```python
from build123d import *

# Parameters (mm, degrees)
ESQUISSE1_R                  = 5
BOSS_EXTRU_1_DEPTH           = 1280
ESQUISSE2_R                  = 15
BOSS_EXTRU_2_DEPTH           = 500
ESQUISSE3_R                  = 10
BOSS_EXTRU_3_DEPTH           = 400
CHANFREIN1_SIZE              = 10
CHANFREIN1_SIZE_2            = 43.314758743
ENL_V_MAT_EXTRU_1_DEPTH      = 1281.175769182
ENL_V_MAT_EXTRU_1_DEPTH_BACK = 1281.175769182
ESQUISSE4_R                  = 4
ESQUISSE5_R                  = 13
ESQUISSE5_R_2                = 9.409989574
BOSS_EXTRU_4_DEPTH           = 10
ESQUISSE7_R                  = 8
ESQUISSE7_R_2                = 4.592937417
BOSS_EXTRU_5_DEPTH           = 10
ESQUISSE6_R                  = 8
ESQUISSE6_R_2                = 4.579122691
BOSS_EXTRU_6_DEPTH           = 10
BOSS_EXTRU_7_START           = 720
BOSS_EXTRU_7_OUTLINE_R       = 13
BOSS_EXTRU_7_OUTLINE_R_2     = 10
BOSS_EXTRU_7_DEPTH           = 10
ESQUISSE8_R                  = 8
ESQUISSE8_R_2                = 4.5
BOSS_EXTRU_8_DEPTH           = 3


# Read off the part's stored shape, not the designer's step: Boss.-Extru.7
with BuildPart() as part:
    # Esquisse1 → Boss.-Extru.1 (new body)
    with BuildSketch(Plane(origin=(0, 0, 0), x_dir=(1, 0, 0), z_dir=(0, 1, 0))):
        with Locations(Location((0, 0, 0), (0, 0, 270))):
            Circle(ESQUISSE1_R)
    extrude(amount=BOSS_EXTRU_1_DEPTH)

    # Esquisse2 → Boss.-Extru.2 (add)
    with BuildSketch(Plane(origin=(0, 0, 0), x_dir=(1, 0, 0), z_dir=(0, 1, 0))):
        with Locations(Location((0, 0, 0), (0, 0, 270))):
            Circle(ESQUISSE2_R)
    extrude(amount=BOSS_EXTRU_2_DEPTH)

    # Esquisse3 → Boss.-Extru.3 (add)
    with BuildSketch(Plane(origin=(0, 500, 0), x_dir=(1, 0, 0), z_dir=(0, 1, 0))):
        with Locations(Location((0, 0, 0), (0, 0, 270))):
            Circle(ESQUISSE3_R)
    extrude(amount=BOSS_EXTRU_3_DEPTH)

    # Chanfrein1
    # the kernel refuses this chamfer: 43.314758743, 10 mm, written as the material it adds along each edge
    with BuildSketch(Plane(origin=(0, 500, 0), x_dir=(0, 0, 1), z_dir=(-1, 0, 0))) as chanfrein1_piece_1_section:
        Polygon((10 + CHANFREIN1_SIZE, 0), (10, CHANFREIN1_SIZE_2), (10, 0), align=None)
    chanfrein1_piece_1 = revolve(axis=Axis((0, 500, 0), (0, 1, 0)), mode=Mode.PRIVATE)
    chanfrein1_piece_1 = chanfrein1_piece_1 & Plane(origin=(0, 533.274352099, 0), x_dir=(0, 0, 1), z_dir=(0, -1, 0)) * Cylinder(15, 174, mode=Mode.PRIVATE)
    add(chanfrein1_piece_1)
    with BuildSketch(Plane(origin=(0, 900, 0), x_dir=(0, 0, 1), z_dir=(1, 0, 0))) as chanfrein1_piece_2_section:
        Polygon((5 + CHANFREIN1_SIZE, 0), (5, -CHANFREIN1_SIZE_2), (5, 0), align=None)
    chanfrein1_piece_2 = revolve(axis=Axis((0, 900, 0), (0, -1, 0)), mode=Mode.PRIVATE)
    chanfrein1_piece_2 = chanfrein1_piece_2 & Plane(origin=(0, 933.283833366, 0), x_dir=(0, 0, 1), z_dir=(0, -1, 0)) * Cylinder(10, 174, mode=Mode.PRIVATE)
    add(chanfrein1_piece_2)

    # Esquisse4 → Enlèv. mat.-Extru.1 (cut, two sides: drawn at the far end of the back side and taken through both)
    with BuildSketch(Plane(origin=(0, 1280, 0), x_dir=(1, 0, 0), z_dir=(0, 1, 0)).offset(-ENL_V_MAT_EXTRU_1_DEPTH_BACK)):
        with Locations(Location((0, 0, 0), (0, 0, 270))):
            Circle(ESQUISSE4_R)
    extrude(amount=ENL_V_MAT_EXTRU_1_DEPTH + ENL_V_MAT_EXTRU_1_DEPTH_BACK, mode=Mode.SUBTRACT)

    # Esquisse5 → Boss.-Extru.4 (add)
    with BuildSketch(Plane(origin=(0, 700, 0), x_dir=(1, 0, 0), z_dir=(0, 1, 0))):
        with Locations(Location((0, 0, 0), (0, 0, 270))):
            Circle(ESQUISSE5_R)
        Circle(ESQUISSE5_R_2, mode=Mode.SUBTRACT)
    extrude(amount=BOSS_EXTRU_4_DEPTH)

    # Esquisse7 → Boss.-Extru.5 (add)
    with BuildSketch(Plane(origin=(0, 1240, 0), x_dir=(1, 0, 0), z_dir=(0, 1, 0))):
        with Locations(Location((0, 0, 0), (0, 0, 270))):
            Circle(ESQUISSE7_R)
        Circle(ESQUISSE7_R_2, mode=Mode.SUBTRACT)
    extrude(amount=BOSS_EXTRU_5_DEPTH)

    # Esquisse6 → Boss.-Extru.6 (add)
    with BuildSketch(Plane(origin=(0, 1000, 0), x_dir=(1, 0, 0), z_dir=(0, 1, 0))):
        with Locations(Location((0, 0, 0), (0, 0, 270))):
            Circle(ESQUISSE6_R)
        Circle(ESQUISSE6_R_2, mode=Mode.SUBTRACT)
    extrude(amount=BOSS_EXTRU_6_DEPTH)

    # Boss.-Extru.7 outline → Boss.-Extru.7 (add)
    with BuildSketch(Plane(origin=(0, 0, 0), x_dir=(1, 0, 0), z_dir=(0, 1, 0)).offset(BOSS_EXTRU_7_START)):
        Circle(BOSS_EXTRU_7_OUTLINE_R)
        Circle(BOSS_EXTRU_7_OUTLINE_R_2, mode=Mode.SUBTRACT)
    extrude(amount=BOSS_EXTRU_7_DEPTH)

    # Esquisse8 → Boss.-Extru.8 (add)
    with BuildSketch(Plane(origin=(0, 1265, 0), x_dir=(1, 0, 0), z_dir=(0, 1, 0))):
        with Locations(Location((0, 0, 0), (0, 0, 270))):
            Circle(ESQUISSE8_R)
        Circle(ESQUISSE8_R_2, mode=Mode.SUBTRACT)
    extrude(amount=BOSS_EXTRU_8_DEPTH)


solid = part.part
```
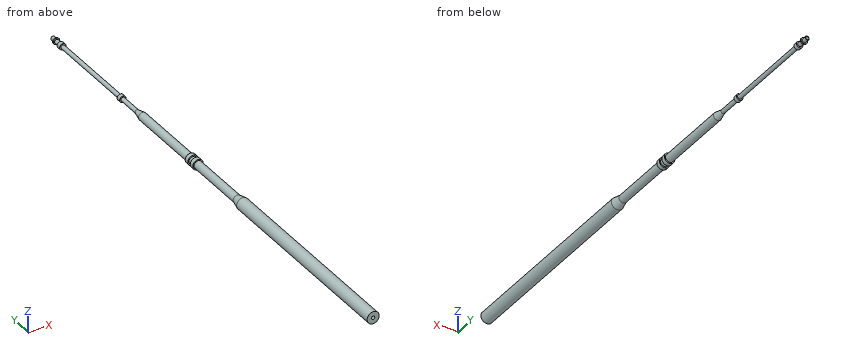
CAD build for the part. Positions are in the model's coordinates, mm. Coordinates: 2 decimals unless noted, no trailing zeros. Write each loop counter-clockwise with the first axis right and the second up, starting at its lowest first coordinate (ties: lowest second). Pieces come first, ordered by that corner, then holes. Notation, with made-up numbers: (-33.75, -30) -> (-2.75, -30) arc R21 cw to (-2.75, 9) -> close; hole circle Ø2 at (60.25, 19.5). An arc over 180 degrees is marked (long way). Return JSON: item names as keys, results as strings. Group by question number.
Q1. Cut at B-B, the plane y = 767. Give the cut face in (x, z).
Q2. Cut at A-A, the plane y = 296. Give the cut face in (x, z).
Q3. Flat gauge pins, fed straight in: pin 1 (13 mm diameter, centred on x = 0, z = 0, fed in from -Y); pin 2 (8 mm diameter, centred on x = 8.5, z = 7, fed in from +Y); pin 3 (10 mm diameter, centred on x = 9.5, y = 324.5, fed in from -Z); pin 4 (4 mm diameter, centred on x = -10, y = 611, fed in from +Z). Where does each tip first touch, or does it go through?
Q4. Drill centre lines: line 1 (X direction, y = 930, z = 0); line 2 (Z direction, x = 1, y = 205); line 3 (X direction, y = 993, z = 0). Where is each one in solid material? Low to high.
Returned:
{
 "1": {"outline": "circle Ø20 at (0, 0); hole circle Ø8 at (0, 0)"},
 "2": {"outline": "circle Ø30 at (0, 0); hole circle Ø8 at (0, 0)"},
 "3": {"pin 1": "stops at y = 0", "pin 2": "stops at y = 1268", "pin 3": "stops at z = -14.31", "pin 4": "stops at z = 6"},
 "4": {"line 1": "x = -8.07 to -4, 4 to 8.07", "line 2": "z = -14.97 to -3.87, 3.87 to 14.97", "line 3": "x = -5 to -4, 4 to 5"}
}
